Input: part model. Units: mm. Frame: model coordinates. Face numbers are marked on the shaded views. Give positions to 0.01 mm unless a question says otherwise; leave off trailing zeros. Loops run counter-clockwise (first coordinate to the right, second up) from the corner with the lowest first, then second, coordinate; pieces in that order, holes last. Notation, with made-up numbers: (-38.75, -17.5) - (-13.75, -17.5) arc R26 cw to (-13.75, 2.5) - close; hole circle Ø8 at (-19, 88.25). An arc over 180 degrees is marked (long way). Answer as a JSON object with one key per item and string values.
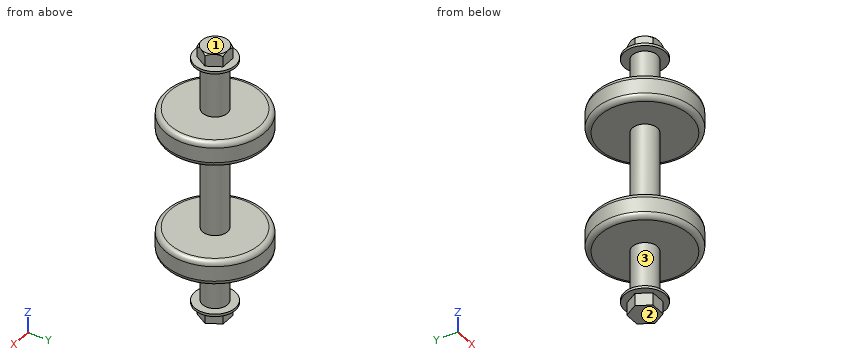
from build123d import *

# Parameters (mm, degrees)
SKETCH2_R           = 25
BOSS_EXTRUDE1_DEPTH = 246.875
SKETCH3_R           = 100
BOSS_EXTRUDE2_DEPTH = 50
FILLET1_R           = 10
SKETCH4_R           = 40.935
BOSS_EXTRUDE3_DEPTH = 5
BOSS_EXTRUDE4_DEPTH = 25
SKETCH6_R           = 40.935
SKETCH6_R_2         = 26.31
CUT_EXTRUDE1_DEPTH  = 25
CUT_EXTRUDE1_TAPER  = 45


with BuildPart() as part:
    # Sketch2 → Boss-Extrude1 (new, symmetric)
    with BuildSketch(Plane.XY):
        with Locations(Location((0, 0, 0), (0, 0, 180))):
            Circle(SKETCH2_R)
    extrude(amount=BOSS_EXTRUDE1_DEPTH, both=True)

    # Sketch3 → Boss-Extrude2 (add)
    with BuildSketch(Plane.XY.offset(146.875)):
        Circle(SKETCH3_R)
    boss_extrude2 = extrude(amount=-BOSS_EXTRUDE2_DEPTH)

    # Mirror1: Boss-Extrude2 across plane
    add(boss_extrude2.mirror(Plane.XY))

    # Fillet1
    fillet1_edges = [part.edges().sort_by_distance(p)[0] for p in [
        (-100, 0, -146.875),
        (-100, 0, -96.875),
        (-100, 0, 96.875),
        (-100, 0, 146.875),
    ]]
    fillet(fillet1_edges, radius=FILLET1_R)

    # Sketch4 → Boss-Extrude3 (add)
    with BuildSketch(Plane.XY.offset(246.875)):
        Circle(SKETCH4_R)
    boss_extrude3 = extrude(amount=BOSS_EXTRUDE3_DEPTH)

    # Sketch5 → Boss-Extrude4 (add)
    with BuildSketch(Plane.XY.offset(251.875)):
        Polygon((30.380171165, 0), (15.190085582, 26.31), (-15.190085582, 26.31), (-30.380171165, 0), (-15.190085582, -26.31), (15.190085582, -26.31), align=None)
    boss_extrude4 = extrude(amount=BOSS_EXTRUDE4_DEPTH)

    # Sketch6 → Cut-Extrude1 (cut)
    with BuildSketch(Plane.XY.offset(276.875)):
        Circle(SKETCH6_R)
        Circle(SKETCH6_R_2, mode=Mode.SUBTRACT)
    extrude(amount=-CUT_EXTRUDE1_DEPTH, taper=CUT_EXTRUDE1_TAPER, mode=Mode.SUBTRACT)

    # Mirror2: Boss-Extrude3, Boss-Extrude4 across plane
    add(boss_extrude3.mirror(Plane.XY))
    add(boss_extrude4.mirror(Plane.XY))


solid = part.part
Item 1: Cut plane A-A (z = -77.5). Return loops of the section in (x, y), then the cut area to 3 significant figures.
Geometry check:
{"outline": "circle Ø50 at (0, 0)", "area": "1,960 mm2"}
Item 2: Mould query, pull axis Z, two halves, no side actions, for the marked faces 1, 2 and 3. Classes: released by +Z, released by -Z, zero draft, split by the parting line, or undercut.
Geometry check:
{"face 1": "released by +Z", "face 2": "released by -Z", "face 3": "undercut"}
Item 3: Material intervals for line 1 (Z direction, x = -25.5, y = 18) (3 decimals); line 2 (Z direction, x = -89, y = 6) (3 decimals); line 3 (Z direction, x = -82, y = -40), sorted ascending. Write a range as [from, to].
Geometry check:
{"line 1": "z = [-251.875, -246.875], [-146.875, -96.875], [96.875, 146.875], [246.875, 251.875]", "line 2": "z = [-146.875, -96.875], [96.875, 146.875]", "line 3": "z = [-146.8, -96.95], [96.95, 146.8]"}
Item 4: Contact query for flat-ended pins moving along their axis: P1, Ø7.5, axis at x = 5.5, z = 263, coming from the +Y side; P2, Ø12.5, axis at x = 5, z = -260, coming from the -Y side; P3, Ø8, axis at x = 51, y = -59.5, coming from the -Z side (3 decimals). Output: stop coordinate, or through.
Geometry check:
{"P1": "stops at y = 26.31", "P2": "stops at y = -26.31", "P3": "stops at z = -146.875"}
